Check sheet for the modelled part. Datum: model origin and axes. Units: mm. A direction names the side the tool comes from. Coordinates: 2 decimals unless noted, no trailing zeros. Order: outer loops, then holes, each group sorted by start corner. A loop starts at its lowest first (then second) coordinate and runs counter-clockwise, first axis right, second up.
Autodesk Fusion 360 part; units mm, degrees
sketch "Sketch1" plane through (0, 0, 0) normal (0, 1, 0) x (1, 0, 0)
  circle A0 centre (16.6339, -3.4008) radius 2.5
  line L0 (13.0339, 6.0992) -> (13.0339, 6.5992)
  line L1 (6.6339, 0.1992) -> (7.1339, 0.1992)
  line L2 (6.6339, 0.1992) -> (7.1339, 0.1992)
  line L3 (10.0732, 2.0992) -> (8.4339, 2.0992)
  line L4 (11.1339, 4.7992) -> (11.1339, 3.1598)
  line L5 (13.5339, 4.7992) -> (13.5339, 6.0992)
  line L6 (20.2339, 6.5992) -> (20.2339, 6.0992)
  line L7 (19.7339, 6.0992) -> (19.7339, 4.7992)
  line L8 (22.1339, 4.7992) -> (19.7339, 4.7992)
  line L9 (13.5339, 4.7992) -> (11.1339, 4.7992)
  line L10 (20.2339, 6.0992) -> (19.7339, 6.0992)
  line L11 (13.5339, 6.0992) -> (13.0339, 6.0992)
  line L12 (25.1339, 6.5992) -> (20.2339, 6.5992)
  line L13 (13.0339, 6.5992) -> (8.1339, 6.5992)
  line L14 (22.1339, 3.1598) -> (22.1339, 4.7992)
  line L15 (24.8339, 2.0992) -> (23.1945, 2.0992)
  line L16 (26.1339, 0.1992) -> (26.6339, 0.1992)
  line L17 (26.1339, 0.1992) -> (26.6339, 0.1992)
  line L18 (22.1339, 0.1992) -> (22.1339, 0.2882)
  line L19 (24.8339, -0.3008) -> (26.1339, -0.3008)
  line L20 (24.8339, -0.3008) -> (26.1339, -0.3008)
  line L21 (24.8339, -8.9008) -> (24.8339, -6.5008)
  line L22 (24.8339, -0.3008) -> (24.8339, 2.0992)
  line L23 (24.8339, -0.3008) -> (24.8339, 2.0992)
  line L24 (26.1339, -7.0008) -> (26.1339, -6.5008)
  line L25 (26.1339, -0.3008) -> (26.1339, 0.1992)
  line L26 (26.6339, -11.9008) -> (26.6339, -7.0008)
  line L27 (26.6339, 0.1992) -> (26.6339, 5.0992)
  line L28 (20.5339, -5.4117) -> (20.5339, -1.3899)
  line L29 (22.1339, 3.1598) -> (20.059, 1.085)
  line L30 (13.2087, 1.085) -> (11.1339, 3.1598)
  line L31 (12.7339, -1.3899) -> (12.7339, -5.4117)
  line L32 (11.1339, 0.1992) -> (11.2666, 0.1992)
  line L33 (18.6448, 0.4992) -> (14.623, 0.4992)
  line L34 (7.1339, -0.3008) -> (8.4339, -0.3008)
  line L35 (16.6339, -3.4008) -> (14.8661, -1.6331) construction
  line L36 (12.7339, 0.4992) -> (6.6339, 6.5992) construction
  line L37 (6.6339, 6.5992) -> (12.7339, 0.4992) construction
  line L38 (13.5339, -1.3615) -> (13.5339, -1.3216)
  line L39 (21.1197, 0.0243) -> (23.1945, 2.0992)
  line L40 (20.059, -7.8866) -> (22.1339, -9.9615)
  line L41 (14.8661, -1.6331) -> (17.1642, -3.9311) construction
  line L42 (26.6339, 6.5992) -> (16.1035, -3.9311) construction
  line L43 (15.0967, -3.8773) -> (14.9766, -3.9974)
  line L44 (15.854, -3.1201) -> (15.8242, -3.1498)
  line L45 (13.0339, -0.9862) -> (13.0339, -0.8615)
  line L46 (10.0732, 2.0992) -> (12.1481, 0.0243)
  line L47 (20.2339, -4.5168) -> (20.2339, -4.6968)
  line L48 (11.1339, -9.9615) -> (11.1339, -11.6008)
  line L49 (8.4339, 2.0992) -> (8.4339, -0.3008)
  line L50 (8.4339, -6.5008) -> (8.4339, -8.9008)
  line L51 (7.1339, 0.1992) -> (7.1339, -0.3008)
  line L52 (7.1339, -0.3008) -> (8.4339, -0.3008)
  line L53 (8.4339, 2.0992) -> (8.4339, -0.3008)
  line L54 (8.4339, -6.5008) -> (8.4339, -8.9008)
  line L55 (6.6339, 5.0992) -> (6.6339, 0.1992)
  line L56 (6.6339, -7.0008) -> (6.6339, -11.9008)
  line L57 (7.1339, -7.0008) -> (6.6339, -7.0008)
  line L58 (8.4339, -6.5008) -> (7.1339, -6.5008)
  line L59 (8.4339, -6.5008) -> (7.1339, -6.5008)
  line L60 (7.1339, -7.0008) -> (6.6339, -7.0008)
  line L61 (7.1339, -6.5008) -> (7.1339, -7.0008)
  line L62 (12.1481, -6.8259) -> (10.0732, -8.9008)
  line L63 (7.1339, -12.9008) -> (6.6339, -13.4008) construction
  line L64 (11.1339, -11.6008) -> (13.5339, -11.6008)
  line L65 (19.7339, -11.6008) -> (22.1339, -11.6008)
  line L66 (13.0339, -12.9008) -> (13.5339, -12.9008)
  line L67 (19.7339, -12.9008) -> (20.2339, -12.9008)
  line L68 (20.2339, -13.4008) -> (25.1339, -13.4008)
  line L69 (8.4339, -8.9008) -> (10.0732, -8.9008)
  line L70 (13.5339, -12.9008) -> (13.5339, -11.6008)
  line L71 (13.0339, -13.4008) -> (13.0339, -12.9008)
  line L72 (26.1339, -6.5008) -> (24.8339, -6.5008)
  line L73 (26.1339, -6.5008) -> (24.8339, -6.5008)
  line L74 (26.6339, -7.0008) -> (26.1339, -7.0008)
  line L75 (26.6339, -7.0008) -> (26.1339, -7.0008)
  line L76 (24.8339, -8.9008) -> (24.8339, -6.5008)
  line L77 (22.1339, -11.6008) -> (22.1339, -9.9615)
  line L78 (23.1945, -8.9008) -> (24.8339, -8.9008)
  line L79 (23.1945, -8.9008) -> (21.1197, -6.8259)
  line L80 (11.1339, -9.9615) -> (13.2087, -7.8866)
  line L81 (14.8661, -5.1686) -> (13.5339, -6.5008) construction
  line L82 (11.1339, -8.9008) -> (8.4339, -11.6008) construction
  line L83 (19.7339, -11.6008) -> (19.7339, -12.9008)
  line L84 (20.2339, -12.9008) -> (20.2339, -13.4008)
  line L85 (18.4016, -5.1686) -> (19.7339, -6.5008) construction
  line L86 (20.5339, -7.3008) -> (26.6339, -13.4008) construction
  line L87 (14.623, -7.3008) -> (18.6448, -7.3008)
  arc A1 (26.6339, 5.0992) -> (25.1339, 6.5992) centre (25.1339, 5.0992) ccw
  arc A2 (8.1339, 6.5992) -> (6.6339, 5.0992) centre (8.1339, 5.0992) ccw
  arc A3 (6.6339, -11.9008) -> (8.1339, -13.4008) centre (8.1339, -11.9008) ccw
  arc A4 (25.1339, -13.4008) -> (26.6339, -11.9008) centre (25.1339, -11.9008) ccw
  arc A5 (13.2087, 1.085) -> (14.623, 0.4992) centre (14.623, 2.4992) ccw
  arc A6 (18.6448, 0.4992) -> (20.059, 1.085) centre (18.6448, 2.4992) ccw
  arc A7 (21.1197, 0.0243) -> (20.5339, -1.3899) centre (22.5339, -1.3899) ccw
  arc A8 (20.5339, -5.4117) -> (21.1197, -6.8259) centre (22.5339, -5.4117) ccw
  arc A9 (20.059, -7.8866) -> (18.6448, -7.3008) centre (18.6448, -9.3008) ccw
  arc A10 (14.623, -7.3008) -> (13.2087, -7.8866) centre (14.623, -9.3008) ccw
  arc A11 (12.1481, -6.8259) -> (12.7339, -5.4117) centre (10.7339, -5.4117) ccw
  arc A12 (12.7339, -1.3899) -> (12.1481, 0.0243) centre (10.7339, -1.3899) ccw
  line L88 (8.1339, -13.4008) -> (13.0339, -13.4008)
  dimension "d1" = 5
  dimension "d2" = 20
  dimension "d3" = 20
  dimension "d8" = 7.2
  dimension "d10" = 7.2
  dimension "d12" = 7.2
  dimension "d14" = 11
  dimension "d15" = 11
  dimension "d17" = 1.5
  dimension "d18" = 1.5
  dimension "d19" = 2
extrude "Extrude1" add sketch "Sketch1" along normal blind 100
(1) Cross-section at B-B (x = 17.75). Enter the section's corners in (y, z), and give its area (3 significant figures).
Filled in:
outline: (0, -0.5) - (100, -0.5) - (100, 1.16) - (0, 1.16) - close; (0, 5.64) - (100, 5.64) - (100, 7.3) - (0, 7.3) - close
area: 333 mm2
(2) Go/stop test with flat-tipped pins: P1, Ø5, axis at x = 20, y = 23.5, coming from the +Z side; P2, Ø3, axis at x = 18, y = 26, coming from the +Z side; P3, Ø1.5, axis at y = 71.5, z = 3.5, coming from the +X side; P4, Ø0.6, axis at x = 7, y = 64, coming from the -Z side. Record where each tip stops, or that it passes through.
Filled in:
P1: stops at z = 13.4
P2: stops at z = 7.49
P3: stops at x = 20.53
P4: stops at z = -6.35
(3) Release check for a two-part mould opening along X. For faces 1 (the flat face through (23, 49, -6.599)), 2 (the flat face through (26.634, 49, 9)), 3 (the flat face through (22.134, 49, -4)) record: +X half, -X half, draft (parallel to the pull), parting line (faces both ways), or undercut.
Filled in:
face 1: draft
face 2: +X half
face 3: undercut
(4) Cross-section at A-A (z = 2.25). Enter the section's corners in (x, y).
Filled in:
outline: (12.73, 0) - (14.41, 0) - (14.41, 100) - (12.73, 100) - close; (18.85, 0) - (20.53, 0) - (20.53, 100) - (18.85, 100) - close
(5) Thickness scan on probe 1 along Z at (x, y) = (13, 93.5); probe 2 along X at (y, z) = (76.5, 11.5); probe 3 along Z at (x, y) = (16.75, 62). Record the ranges inside material, lowest first.
Filled in:
probe 1: z = -6.6 to -4.8, -1.29 to 8.1, 11.6 to 13.4
probe 2: x = 6.63 to 11.13, 22.13 to 26.63
probe 3: z = -0.5 to 0.9, 5.9 to 7.3
(6) Tool access check on faces 4 (the flat face through (24.834, 49, 8)), 5 (the flat face through (12.734, 49, 3)), 6 (the flat face through (17, 49, -0.499)). Record the directions out of +Z, -Z, +X, -X, +Y, -Y that give a thin tool (end or side, any length) a straight path to the whole face; none if there is none.
Filled in:
face 4: +Y, -Y
face 5: -X, +Y, -Y
face 6: -Z, +Y, -Y
